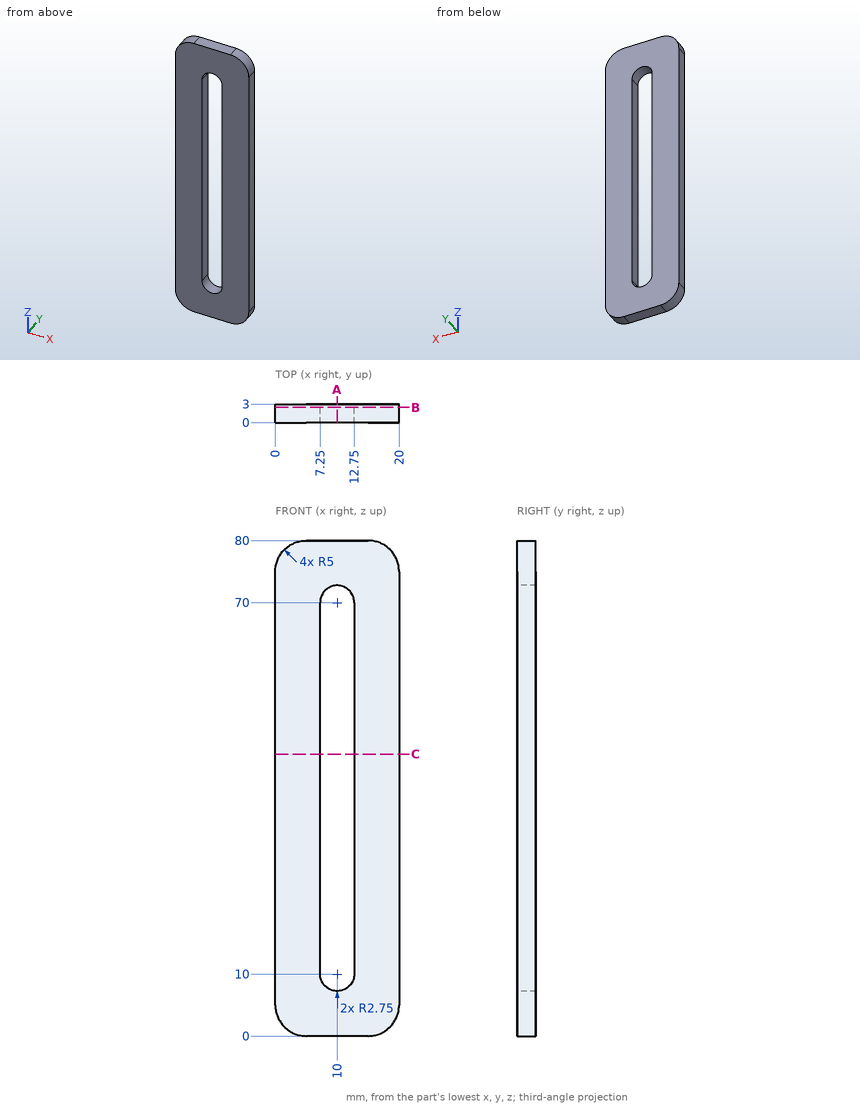
Drawing for the job (mm, zero at the part's lowest x, y, z). Round coordinates to 2 decimals unless told otherwise and drop trailing zeros. Write each loop counter-clockwise with the first axis right and the second up, starting at its lowest first coordinate (ties: lowest second). Pieces come first, ordered by that corner, then holes. Notation, with made-up numbers: M 28.25,83 L 55.25,83 A19 cw 55.25,106 Z; hole C 78,5.5 d4. An arc over 180 degrees is marked long. Answer as a JSON object with one key per item and string values. Group by question number.
(1) Cut at B-B (y = 2.45). Give the cut face in (x, z), and give its area (3 significant figures).
(2) Cut at C-C (z = 45.5). Give the cut face in (x, y).
(3) Cut at A-A (x = 10). Give the cut face in (y, z), and give its area (3 significant figures).
(4) Drill centre lines: L1, parallel to X at y = 2.85, z = 67; L2, parallel to X at y = 0.45, z = 7.5; L3, parallel to Z at x = 9.75, y = 0.25. Where is each one in solid material? Low to high.
Responses:
{
 "1": {"outline": "M 0,5 A5 ccw 5,0 L 15,0 A5 ccw 20,5 L 20,75 A5 ccw 15,80 L 5,80 A5 ccw 0,75 Z; hole M 7.25,10 A2.75 ccw 12.75,10 L 12.75,70 A2.75 ccw 7.25,70 Z", "area": "1,220 mm2"},
 "2": {"outline": "M 0,0 L 7.25,0 L 7.25,3 L 0,3 Z; M 12.75,0 L 20,0 L 20,3 L 12.75,3 Z"},
 "3": {"outline": "M 0,0 L 3,0 L 3,7.25 L 0,7.25 Z; M 0,72.75 L 3,72.75 L 3,80 L 0,80 Z", "area": "43.5 mm2"},
 "4": {"L1": "x = 0 to 7.25, 12.75 to 20", "L2": "x = 0 to 8.85, 11.15 to 20", "L3": "z = 0 to 7.26, 72.74 to 80"}
}
